```python
from build123d import *

# Parameters (mm, degrees)
SKETCH2_R           = 1.7
RESISTOR_BODY_DEPTH = 10
LEAD1_PROFILE_R     = 0.4
SKETCH6_R           = 0.4
LEAD2_DEPTH         = 5.3


with BuildPart() as part:
    # Sketch2 → Resistor Body (new body)
    with BuildSketch(Plane.XY):
        Circle(SKETCH2_R)
    extrude(amount=RESISTOR_BODY_DEPTH)

    # Lead1: sweep along a path in Lead1 Path
    with BuildLine(Plane(origin=(0, 0, 0), x_dir=(1, 0, 0), z_dir=(0, 1, 0))) as lead1_path:
        Line((4, 5.3), (4, -10))
        ThreePointArc((4, -10), (2, -12), (0, -10))
    # Lead1 Profile → Lead1 (sweep)
    with BuildSketch(Plane(origin=(0, 0, 10), x_dir=(-1, 0, 0), z_dir=(0, 0, 1))):
        Circle(LEAD1_PROFILE_R)
    sweep(path=lead1_path.line)

    # Sketch6 → Lead2 (add)
    with BuildSketch(Plane(origin=(0, 0, 0), x_dir=(1, 0, 0), z_dir=(0, 0, -1))):
        Circle(SKETCH6_R)
    extrude(amount=LEAD2_DEPTH)


solid = part.part
```
Source: CAD feature listing. Evaluate the final solid. Frame: model axes, mm. Coordinates: 2 decimals unless noted, no trailing zeros. Write each loop counter-clockwise with the first axis right and the second up, starting at its lowest first coordinate (ties: lowest second). Pieces come first, ordered by that corner, then holes. Notation, with made-up numbers: (55, 82) - (102, 82) arc R20 cw to (102, 115) - close; hole circle Ø11 at (-5, 5.25). An arc over 180 degrees is marked (long way). Answer as a JSON object with one key per item and string values.
Q1. Section query C-C, the plane y = -1. Output: boundary loops of the cut face in (x, z).
Ans:
{"outline": "(-1.37, 0) - (1.37, 0) - (1.37, 10) - (-1.37, 10) - close"}
Q2. First-contact query: pin 1 Ø1.5 at (y, z) = (0.5, 5) entering from -X; pin 2 Ø1.5 at (x, z) = (3, 8) entering from +Y; pin 3 Ø1.5 at (x, y) = (0.5, -0.5) entering from +Z (3 decimals). Flat tips, straight axial feed; report the tip coordinate or a pass-through.
Ans:
{"pin 1": "stops at x = -1.7", "pin 2": "stops at y = 0.31", "pin 3": "stops at z = 12.225"}
Q3. Draft query along Y for faces 1 (the cylindrical face through (-0.37, -1.66, 4.93)), 2 (the flat face through (0.4, -0.4, 10)). Return one class per face: released by +Y, released by -Y, zero draft, split by the parting line, or undercut.
Ans:
{"face 1": "split by the parting line", "face 2": "zero draft"}
Q4. Section query A-A, the plane z = 2.25. Output: boundary loops of the cut face in (x, y).
Ans:
{"outline": "circle Ø3.4 at (0, 0); circle Ø0.8 at (4, 0)"}
Q5. Material intervals for line 1 (Z direction, x = -0.75, y = 0.9); line 2 (X direction, y = 0.2, z = -3.5); line 3 (Y direction, x = -1, z = 6.25), sorted ascending. Write a range as [from, to].
Ans:
{"line 1": "z = [0, 10]", "line 2": "x = [-0.35, 0.35], [3.65, 4.35]", "line 3": "y = [-1.37, 1.37]"}
Q6. Section query B-B, the plane y = 0. Output: boundary loops of the cut face in (x, z).
Ans:
{"outline": "(-1.7, 0) - (-0.4, 0) - (-0.4, -5.3) - (0.4, -5.3) - (0.4, 0) - (1.7, 0) - (1.7, 10) - (0.4, 10) arc R1.6 cw to (3.6, 10) - (3.6, -5.3) - (4.4, -5.3) - (4.4, 10) arc R2.4 ccw to (-0.4, 10) - (-1.7, 10) - close"}
